Autodesk Inventor part; units mm, degrees
ref_plane "YZ Plane" through (0, 0, 0) normal (1, 0, 0) x (0, 1, 0)
ref_plane "XZ Plane" through (0, 0, 0) normal (0, 1, 0) x (-1, 0, 0)
ref_plane "XY Plane" through (0, 0, 0) normal (0, 0, 1) x (1, 0, 0)
sketch "Sketch1" plane through (0, 0, 0) normal (0, 1, 0) x (-1, 0, 0)
  arc A0 (2.4889, -2.6698) -> (-2.4889, -2.6698) centre (0, 0) ccw
  line L0 (2.4889, -2.6698) -> (4.9794, -2.6698)
  line L1 (-4.9794, -2.6698) -> (-2.4889, -2.6698)
  line L2 (-5.65, 0) -> (-5.65, 76)
  line L3 (5.65, 76) -> (5.65, 0)
  arc A1 (-2.4889, 154.6698) -> (2.4889, 154.6698) centre (0, 152) ccw
  line L4 (2.4889, 154.6698) -> (4.9794, 154.6698)
  line L5 (-4.9794, 154.6698) -> (-2.4889, 154.6698)
  line L6 (-5.65, 152) -> (-5.65, 76)
  line L7 (5.65, 76) -> (5.65, 152)
  arc A2 (4.9794, -2.6698) -> (5.65, 0) centre (0, 0) ccw
  arc A3 (-5.65, 0) -> (-4.9794, -2.6698) centre (0, 0) ccw
  arc A4 (-4.9794, 154.6698) -> (-5.65, 152) centre (0, 152) ccw
  arc A5 (5.65, 152) -> (4.9794, 154.6698) centre (0, 152) ccw
  dimension "d5" = 7.3
  dimension "d7" = 76
extrude "Extrusion1" add sketch "Sketch1" along normal blind 3
properties part number "Holder 2"
Could you check a few things on this model? Use its own coordinates, in mm. Round coordinates to 2 decimals unless told otherwise and drop trailing zeros. Order: outer loops, then holes, each group sorted by start corner. A loop starts at its lowest first (then second) coordinate and runs counter-clockwise, first axis right, second up. Notation, with made-up numbers: M 16.5,72.5 L 33.5,72.5 A26 ccw 33.5,108.5 Z; hole C 2,59 d10. An arc over 180 degrees is marked long. One line per question, with ' | ' between items. Start each with the question number.
(1) Suppose I cut it at A-A on y = 0.85. List the corners of the cut face in (x, z) for me, then the cut area to 3 significant figures.
(2) For P1, Ø6, axis at x = 0, z = 152, coming from the +Y side; P2, Ø1, axis at x = 1.5, y = 1.5, coming from the +Z side, each with a flat end and sliding along its axis, tell me the tip position at first contact or that it passes through.
(3) Please list where these lines run through material, in increasing order: line 1 along X through (y, z) = (1.05, 152); line 2 along Z through (x, y) = (-3, 0.5); line 3 along Z through (x, y) = (-1.5, 1.55).
(4) Thinking about a two-plate mould opening in Z: for faces 1 (the face through (0.12, 1.48, 3.65)), 2 (the face through (-4, 1, -2.67)), 3 (the face through (-5.65, 1, 77)), which applies, +Z half, -Z half, draft (parallel to the pull), parting line (faces both ways), or undercut?
(5) Suppose I cut it at B-B on x = 0. List the corners of the cut face in (y, z) for me.
Geometry results:
1) outline: M -5.65,0 A5.65 ccw -4.98,-2.67 L -2.49,-2.67 A3.65 cw long 2.49,-2.67 L 4.98,-2.67 A5.65 ccw 5.65,0 L 5.65,152 A5.65 ccw 4.98,154.67 L 2.49,154.67 A3.65 cw long -2.49,154.67 L -4.98,154.67 A5.65 ccw -5.65,152 Z | area: 1,700 mm²
2) P1: through | P2: z = 148.95
3) line 1: -5.65 to -3.65, 3.65 to 5.65 | line 2: -2.67 to -2.08, 2.08 to 149.92, 154.08 to 154.67 | line 3: 3.33 to 148.67
4) face 1: undercut | face 2: -Z half | face 3: draft
5) outline: M 0,3.65 L 3,3.65 L 3,148.35 L 0,148.35 Z
